```python
from build123d import *

# Parameters (mm, degrees)
EXTRUDE_1_DEPTH       = 20
CUT_EXTRUDE_1_DEPTH   = 39.678159
SKETCH_5_R            = 3
CUT_EXTRUDE_2_DEPTH   = 3
SKETCH_6_W            = 10
SKETCH_6_H            = 12
CUT_EXTRUDE_3_DEPTH   = 46.650849
F_3_0MM_1_D           = 3
F_3_0MM_1_CSINK_D     = 3.05
F_3_0MM_1_CSINK_ANGLE = 90
CHAMFER_2_SIZE        = 2
CUT_EXTRUDE_START     = -3
SKETCH_9_R            = 3
CUT_EXTRUDE_5_DEPTH   = 3
SKETCH_10_W           = 5
SKETCH_10_H           = 20
EXTRUDE_2_DEPTH       = 11
CHAMFER_3_SIZE        = 3
CHAMFER_4_SIZE        = 1


with BuildPart() as part:
    # 草图1 → 凸台-拉伸1 (new body)
    with BuildSketch(Plane.XY):
        with BuildLine():
            Line((0, 14), (-30, 14))
            Line((-30, 14), (-30, -14))
            Line((-30, -14), (0, -14))
            ThreePointArc((0, -14), (14, 0), (0, 14))
        make_face()
    extrude(amount=EXTRUDE_1_DEPTH)

    # 草图3 → 切除-拉伸1 (cut, through all)
    with BuildSketch(Plane(origin=(0, 0, 0), x_dir=(-1, 0, 0), z_dir=(0, 0, -1))):
        with BuildLine():
            Line((-3, 0), (1.5, -2.598076))
            ThreePointArc((1.5, -2.598076), (1.5, 2.598076), (-3, 0))
        make_face()
    extrude(amount=-CUT_EXTRUDE_1_DEPTH, mode=Mode.SUBTRACT)

    # 草图5 → 切除-拉伸2 (cut)
    with BuildSketch(Plane(origin=(0, 0, 0), x_dir=(-1, 0, 0), z_dir=(0, 0, -1))):
        Circle(SKETCH_5_R)
    extrude(amount=-CUT_EXTRUDE_2_DEPTH, mode=Mode.SUBTRACT)

    # 草图6 → 切除-拉伸3 (cut, through all)
    with BuildSketch(Plane.XZ.offset(14)):
        with Locations((-25, 10)):
            Rectangle(SKETCH_6_W, SKETCH_6_H)
    extrude(amount=-CUT_EXTRUDE_3_DEPTH, mode=Mode.SUBTRACT)

    # Ø3.0mm 暗销孔1 (through all)
    with Locations(Plane(origin=(-25, 6, 0), x_dir=(-1, 0, 0), z_dir=(0, 0, -1))):
        with Locations((0, 0), (0, -12)):
            CounterSinkHole(F_3_0MM_1_D / 2, F_3_0MM_1_CSINK_D / 2, counter_sink_angle=F_3_0MM_1_CSINK_ANGLE)

    # 倒角2
    chamfer_2_edges = [part.edges().sort_by_distance(p)[0] for p in [
        (-30, -14, 2),
        (-30, 14, 2),
        (-30, -14, 18),
        (-30, 14, 18),
    ]]
    chamfer(chamfer_2_edges, length=CHAMFER_2_SIZE)

    # 草图9 → 切除-拉伸5 (cut)
    with BuildSketch(Plane.XY.offset(20).offset(CUT_EXTRUDE_START)):
        with Locations(Location((0, 0, 0), (0, 0, 180))):
            Circle(SKETCH_9_R)
    extrude(amount=CUT_EXTRUDE_5_DEPTH, mode=Mode.SUBTRACT)

    # 草图10 → 凸台-拉伸2 (add)
    with BuildSketch(Plane.XZ.offset(14)):
        with Locations((-17.5, 10)):
            Rectangle(SKETCH_10_W, SKETCH_10_H)
    extrude(amount=EXTRUDE_2_DEPTH)

    # 倒角3
    chamfer_3_edges = [part.edges().sort_by_distance(p)[0] for p in [
        (-17.5, -25, 0),
        (-17.5, -25, 20),
    ]]
    chamfer(chamfer_3_edges, length=CHAMFER_3_SIZE)

    # 倒角4
    chamfer_4_edges = [part.edges().sort_by_distance(p)[0] for p in [
        (-2.598076, -1.5, 20),
        (1.5, 2.598076, 0),
    ]]
    chamfer(chamfer_4_edges, length=CHAMFER_4_SIZE)


solid = part.part
```
CAD build for the part. Positions are in the model's coordinates, mm. A direction names the side the tool comes from. Round coordinates to 2 decimals unless told otherwise and drop trailing zeros. Write each loop counter-clockwise with the first axis right and the second up, starting at its lowest first coordinate (ties: lowest second). Pieces come first, ordered by that corner, then holes. Notation, with made-up numbers: (4, 77.25) - (41, 77.25) arc R22 cw to (41, 83.25) - close; hole circle Ø1 at (16, 47). An arc over 180 degrees is marked (long way). Return JSON: item names as keys, results as strings. Group by question number.
Item 1: Band-saw the part on C-C on z = 12.25. List the corners of the cut face in (x, y), plus the area to 3 significant figures.
Item 2: Probe probe 1 along Y at (x, z) = (-25, 3.1); probe 2 along Z at (x, y) = (-28, 3); probe 3 along Y at (x, z) = (-10.5, 11.75). List the from-to ranges inside material, lowest first.
Item 3: Flat gauge pins, fed straight in: pin 1 Ø3 at (y, z) = (-15, 8.5) entering from -X; pin 2 Ø4 at (x, y) = (-20.5, 9) entering from -Z; pin 3 Ø3.5 at (y, z) = (-21, 8.5) entering from +X; pin 4 Ø10 at (x, z) = (0.5, 10.5) entering from -Y. Where does each tip first touch, or does it go through?
Item 4: Band-saw the part on B-B on y = -6. List the corners of the cut face in (x, z) (3 decimals).
Item 5: 3-axis set-ups, long thin cutter, end or side, ignore diameter. For faces 4 (the face through (-24, -14, 2)), 5 (the face through (1, -2, 3)), 6 (the face through (0.78, -1.28, 9.9)): which of +Z, -Z, +X, -X, +Y, -Y reach the whole face in a straight line?
Item 6: Band-saw the part on A-A on x = -25. List the corners of the cut face in (y, z) (3 decimals), plus the area to 3 significant figures.
Item 7: Band-saw the part on D-D on y = -10. List the corners of the cut face in (x, z).
Item 8: Mould opens along Z. For faces 1 (the face through (-18, -24, 18)), 2 (the face through (-25, 0, 16)), 3 (the face through (-15, -19, 10)) say: +Z half, -Z half, draft (parallel to the pull), parting line (faces both ways), or undercut.
Resolved:
{
 "1": {"outline": "(-20, -25) - (-15, -25) - (-15, -14) - (0, -14) arc R14 ccw to (0, 14) - (-20, 14) - close; hole (-1.5, -2.6) - (3, 0) arc R3 ccw (long way) to start", "area": "900 mm²"},
 "2": {"probe 1": "y = -14 to -7.5, -4.5 to 4.5, 7.5 to 14", "probe 2": "z = 0 to 4, 16 to 20", "probe 3": "y = -14 to 14"},
 "3": {"pin 1": "stops at x = -20", "pin 2": "stops at z = 0", "pin 3": "stops at x = -15", "pin 4": "stops at y = -14"},
 "4": {"outline": "(-30, 0) - (-26.525, 0) - (-26.5, 0.025) - (-26.5, 4) - (-30, 4) - close; (-30, 16) - (-26.5, 16) - (-26.5, 20) - (-30, 20) - close; (-23.5, 0.025) - (-23.475, 0) - (12.649, 0) - (12.649, 20) - (-23.5, 20) - (-23.5, 16) - (-20, 16) - (-20, 4) - (-23.5, 4) - close"},
 "5": {"face 4": "+Z, -Z, -X, -Y", "face 5": "-Z", "face 6": "+Z, -Z"},
 "6": {"outline": "(-14, 0) - (-7.525, 0) - (-7.5, 0.025) - (-7.5, 4) - (-14, 4) - close; (-14, 16) - (-7.5, 16) - (-7.5, 20) - (-14, 20) - close; (-4.5, 0.025) - (-4.475, 0) - (4.475, 0) - (4.5, 0.025) - (4.5, 4) - (-4.5, 4) - close; (-4.5, 16) - (4.5, 16) - (4.5, 20) - (-4.5, 20) - close; (7.5, 0.025) - (7.525, 0) - (14, 0) - (14, 4) - (7.5, 4) - close; (7.5, 16) - (14, 16) - (14, 20) - (7.5, 20) - close", "area": "176 mm²"},
 "7": {"outline": "(-30, 0) - (9.8, 0) - (9.8, 20) - (-30, 20) - (-30, 16) - (-20, 16) - (-20, 4) - (-30, 4) - close"},
 "8": {"face 1": "+Z half", "face 2": "undercut", "face 3": "draft"}
}
